from build123d import *

# Parameters (mm, degrees)
F1_DEPTH = 30
F4_DEPTH = 60


with BuildPart() as f1:
    # F0 (on Right) → F1 (new body)
    with BuildSketch(Plane.YZ):
        Polygon((15.664, -27.1308438498), (31.328, 0), (15.664, 27.1308438498), (-15.664, 27.1308438498), (-31.328, 0), (-15.664, -27.1308438498), align=None)
    extrude(amount=F1_DEPTH)



with BuildPart() as f4:
    # F3 (on offset) → F4 (new body)
    with BuildSketch(Plane.YZ.offset(-24.5)):
        Polygon((15.8121267025, -27.0447819948), (31.3275315985, 0.1713124148), (15.515404896, 27.2160944096), (-15.8121267025, 27.0447819948), (-31.3275315985, -0.1713124148), (-15.515404896, -27.2160944096), align=None)
    extrude(amount=-F4_DEPTH)


with BuildPart() as f1_1:
    add(f1.part)

    add(f4.part)  # F8 merges F4
    # F6 (on Right) → F8 section 0
    with BuildSketch(Plane.YZ, mode=Mode.PRIVATE) as f8_s0:
        Polygon((15.664, -27.1308438498), (31.328, 0), (15.664, 27.1308438498), (-15.664, 27.1308438498), (-31.328, 0), (-15.664, -27.1308438498), align=None)
    loft([f8_s0.sketch, Vertex(-24.5, 0, 0)])

    # F7 (on offset) → F9 section 0
    with BuildSketch(Plane.YZ.offset(-24.5), mode=Mode.PRIVATE) as f9_s0:
        Polygon((15.664, -27.1308438498), (31.328, 0), (15.664, 27.1308438498), (-15.664, 27.1308438498), (-31.328, 0), (-15.664, -27.1308438498), align=None)
    loft([f9_s0.sketch, Vertex(0, 0, 0)])

    # F10: F1 across plane


with BuildPart() as f1_2:
    add(f1_1.part)
    add(f1_1.part.mirror(Plane(origin=(-84.5, 0, 0), x_dir=(0, 1, 0), z_dir=(-1, 0, 0))))


solid = f1_2.part
Verification items for the finished model (mm, model axes). A direction names the side the tool comes from. Give positions to 0.01 mm unless a question says otherwise; leave off trailing zeros. Write each loop counter-clockwise with the first axis right and the second up, starting at its lowest first coordinate (ties: lowest second). Pieces come first, ordered by that corner, then holes. Notation, with made-up numbers: M 9,-23.75 L 68,-23.75 A21 cw 68,10.25 Z; hole C 69.5,23 d7. An arc over 180 degrees is marked long. Write item = value, one per line.
(1) Sectioned sample at B-B (y = 21). Record the cut outline in (x, z), then the cut area to 3 significant figures.
Found:
outline = M -199,-17.89 L -169,-17.89 L -160.92,0 L -169,17.89 L -199,17.89 Z; M -152.58,0 L -144.5,-17.89 L -144.5,-17.94 L -24.5,-17.94 L -24.5,-17.89 L -16.42,0 L -24.5,17.89 L -24.5,17.84 L -144.5,17.84 L -144.5,17.89 Z; M -8.08,0 L 0,-17.89 L 30,-17.89 L 30,17.89 L 0,17.89 Z
area = 7,020 mm2
(2) Access from +Z, -Z, +X, -X, +Y, -Y to the whole of each face (thin tool, end or side, straight path). Record for faces 3 (the face through (-164.15, 18.735, -11.07)), 4 (the face through (-164.15, 0.22, 21.76)).
Found:
face_3 = -Z, +Y
face_4 = +Z, +Y, -Y
(3) Sectioned sample at C-C (z = 21.5). Record the cut outline in (x, y), then the cut area to 3 significant figures.
Found:
outline = M -199,-18.91 L -169,-18.91 L -163.92,-12.41 L -163.92,12.41 L -169,18.91 L -199,18.91 Z; M -149.58,-12.41 L -144.5,-18.91 L -144.5,-18.97 L -24.5,-18.97 L -24.5,-18.91 L -19.42,-12.41 L -19.42,12.41 L -24.5,18.91 L -24.5,18.86 L -144.5,18.86 L -144.5,18.91 L -149.58,12.41 Z; M -5.08,-12.41 L 0,-18.91 L 30,-18.91 L 30,18.91 L 0,18.91 L -5.08,12.41 Z
area = 7,450 mm2
(4) Sectioned sample at A-A (x = -90.5). Record the cut outline in (y, z), then the cut area to 3 significant figures.
Found:
outline = M -31.33,-0.17 L -15.52,-27.22 L 15.81,-27.04 L 31.33,0.17 L 15.52,27.22 L -15.81,27.04 Z
area = 2,550 mm2
(5) Draft check along X on faces 1 (the face through (-164.15, 18.955, 10.69)), 2 (the face through (-184, 0, 27.131)). Enter one of: released by +X, released by -X, zero draft, split by the parting line, or undercut.
Found:
face_1 = undercut
face_2 = zero draft
(6) Go/stop test with flat-tipped pins: pin 1 Ø15 at (x, y) = (8.5, 6.5) entering from -Z; pin 2 Ø1 at (x, y) = (-25, 21) entering from +Z; pin 3 Ø2 at (x, z) = (-86.5, 10.5) entering from +Y. Record where each tip stops, or that it passes through.
Found:
pin_1 = -27.13
pin_2 = 18.69
pin_3 = 25.87
(7) Sectioned sample at D-D (z = 6.5). Record the cut outline in (x, y).
Found:
outline = M -199,-27.58 L -169,-27.58 L -156.75,-11.91 L -144.5,-27.58 L -144.5,-27.52 L -24.5,-27.52 L -24.5,-27.58 L -12.25,-11.91 L 0,-27.58 L 30,-27.58 L 30,27.58 L 0,27.58 L -12.25,11.91 L -24.5,27.58 L -24.5,27.63 L -144.5,27.63 L -144.5,27.58 L -156.75,11.91 L -169,27.58 L -199,27.58 Z
(8) Material ranges on line 1 (X direction, y = 19, z = 1.5); line 2 (X direction, y = -4, z = 20.5); line 3 (Z direction, x = -99.5, y = 11), recorded low to high.
Found:
line_1 = -199 to -160.04, -153.46 to -15.54, -8.96 to 30
line_2 = -199 to -163.01, -150.49 to -18.51, -5.99 to 30
line_3 = -27.07 to 27.19
